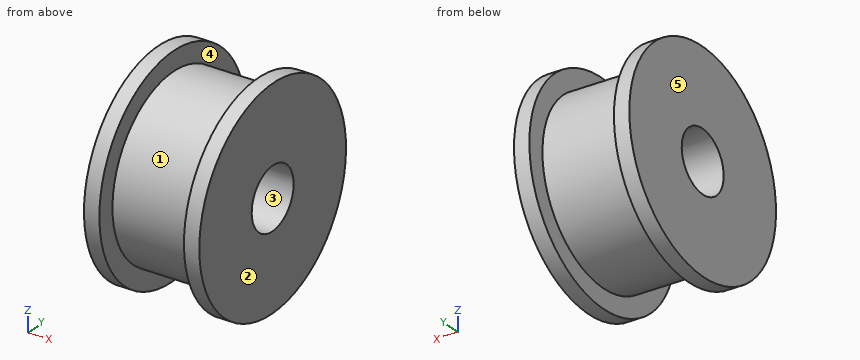
from build123d import *

# Parameters (mm, degrees)
SKETCH1_R           = 14
SKETCH1_R_2         = 4
BOSS_EXTRUDE1_DEPTH = 7.5
SKETCH2_OUTSIDE_W   = 38.468
SKETCH2_OUTSIDE_H   = 38.468
SKETCH2_OUTSIDE_R   = 11.5
CUT_EXTRUDE1_DEPTH  = 5.5


with BuildPart() as part:
    # Sketch1 → Boss-Extrude1 (new, symmetric)
    with BuildSketch(Plane(origin=(0, 0, 0), x_dir=(0, 0, -1), z_dir=(1, 0, 0))):
        Circle(SKETCH1_R)
        Circle(SKETCH1_R_2, mode=Mode.SUBTRACT)
    extrude(amount=BOSS_EXTRUDE1_DEPTH, both=True)

    # Sketch2 outside → Cut-Extrude1 (cut, symmetric)
    with BuildSketch(Plane(origin=(0, 0, 0), x_dir=(0, 0, -1), z_dir=(1, 0, 0))):
        Rectangle(SKETCH2_OUTSIDE_W, SKETCH2_OUTSIDE_H)
        Circle(SKETCH2_OUTSIDE_R, mode=Mode.SUBTRACT)
    extrude(amount=CUT_EXTRUDE1_DEPTH, both=True, mode=Mode.SUBTRACT)


solid = part.part
Geometry: final body of the model. Coordinates: model frame, mm. Face numbers are marked on the shaded views. A direction names the side the tool comes from. Give positions to 0.01 mm unless a question says otherwise; leave off trailing zeros. Write each loop counter-clockwise with the first axis right and the second up, starting at its lowest first coordinate (ties: lowest second). Pieces come first, ordered by that corner, then holes. Notation, with made-up numbers: (64.25, 7.25) -> (76.25, 7.25) arc R14 ccw to (76.25, 19.25) -> close; hole circle Ø3 at (33, 89.5). An arc over 180 degrees is marked (long way). Answer as a JSON object with one key per item and string values.
1. Access query for the marked faces 4 and 5. Directions: +Z, -Z, +X, -X, +Y, -Y. A direction counts if a zero-diameter tool reaches every point of the face in a straight line with its end or side. Return the directions, or none.
Ans:
{"face 4": "none", "face 5": "+Z, -Z, -X, +Y, -Y"}
2. Mould query, pull axis X, two halves, no side actions, for the marked faces 1, 2 and 3. Classes: pulls with the +X half, pulls with the -X half, needs draft (parallel to the pull), parting line crosses it, or undercut.
Ans:
{"face 1": "undercut", "face 2": "pulls with the +X half", "face 3": "needs draft"}
3. Contact query for flat-ended pins moving along their axis: pin 1 (3 mm diameter, centred on x = -2, y = -8.5, fed in from -Z); pin 2 (3 mm diameter, centred on x = 1, y = -9, fed in from -Z). Output: stop coordinate, or through.
Ans:
{"pin 1": "stops at z = -9.12", "pin 2": "stops at z = -8.72"}
4. Cut plane A-A on y = 0. Output: boundary loops of the cut face in (x, z), and give its area (3 significant figures).
Ans:
{"outline": "(-7.5, -14) -> (-5.5, -14) -> (-5.5, -11.5) -> (5.5, -11.5) -> (5.5, -14) -> (7.5, -14) -> (7.5, -4) -> (-7.5, -4) -> close; (-7.5, 4) -> (7.5, 4) -> (7.5, 14) -> (5.5, 14) -> (5.5, 11.5) -> (-5.5, 11.5) -> (-5.5, 14) -> (-7.5, 14) -> close", "area": "245 mm^2"}
5. Cut plane D-D on z = 5.25. Output: boundary loops of the cut face in (x, y).
Ans:
{"outline": "(-7.5, -12.98) -> (-5.5, -12.98) -> (-5.5, -10.23) -> (5.5, -10.23) -> (5.5, -12.98) -> (7.5, -12.98) -> (7.5, 12.98) -> (5.5, 12.98) -> (5.5, 10.23) -> (-5.5, 10.23) -> (-5.5, 12.98) -> (-7.5, 12.98) -> close"}
6. Ray query, probe 1 along X at (y, z) = (9, 10.25); probe 2 along Y at (x, z) = (-0.5, 0); probe 3 along Z at (x, y) = (5.25, 0.25). Return the intervals inside material, ascending. Write a range as from..to.
Ans:
{"probe 1": "x = -7.5..-5.5, 5.5..7.5", "probe 2": "y = -11.5..-4, 4..11.5", "probe 3": "z = -11.5..-3.99, 3.99..11.5"}
7. Cut plane C-C on x = 6.25. Output: boundary loops of the cut face in (y, z), and give its area (3 significant figures).
Ans:
{"outline": "circle Ø28 at (0, 0); hole circle Ø8 at (0, 0)", "area": "565 mm^2"}
